```python
from build123d import *

# Parameters (mm, degrees)
SKETCH1_W           = 70.58
SKETCH1_H           = 55.34
SKETCH1_R           = 1.5875
BOSS_EXTRUDE1_DEPTH = 4
SKETCH2_R           = 2.5
CUT_EXTRUDE1_DEPTH  = 6
SKETCH3_R           = 2.5875
SKETCH3_R_2         = 1.5875
SKETCH3_R_3         = 0.9525
BOSS_EXTRUDE2_DEPTH = 3.175


with BuildPart() as part:
    # Sketch1 → Boss-Extrude1 (new, symmetric)
    with BuildSketch(Plane.XY):
        Rectangle(SKETCH1_W, SKETCH1_H)
        with Locations((-20.32, 24.13)):
            Circle(SKETCH1_R, mode=Mode.SUBTRACT)
        with Locations((30.48, 8.89)):
            Circle(SKETCH1_R, mode=Mode.SUBTRACT)
        with Locations((30.48, -19.05)):
            Circle(SKETCH1_R, mode=Mode.SUBTRACT)
        with Locations((-21.59, -24.13)):
            Circle(SKETCH1_R, mode=Mode.SUBTRACT)
    extrude(amount=BOSS_EXTRUDE1_DEPTH, both=True)

    # Sketch2 → Cut-Extrude1 (cut)
    with BuildSketch(Plane(origin=(0, -27.67, 0), x_dir=(1, 0, 0), z_dir=(0, 1, 0))):
        with Locations(Location((30, 0, 0), (0, 0, 270))):
            Circle(SKETCH2_R)
        with Locations(Location((-30, 0, 0), (0, 0, 90))):
            Circle(SKETCH2_R)
    extrude(amount=CUT_EXTRUDE1_DEPTH, mode=Mode.SUBTRACT)

    # Sketch3 → Boss-Extrude2 (add)
    # profile 1 of 4: a face of its own
    with BuildSketch(Plane.XY.offset(4)):
        with Locations(Location((-20.32, 24.13, 0), (0, 0, 180))):
            Circle(SKETCH3_R)
        with Locations((-20.32, 24.13)):
            Circle(SKETCH3_R_2, mode=Mode.SUBTRACT)
    # profile 2 of 4: a face of its own
    with BuildSketch(Plane.XY.offset(4)):
        with Locations(Location((-21.59, -24.13, 0), (0, 0, 180))):
            Circle(SKETCH3_R)
        with Locations((-21.59, -24.13)):
            Circle(SKETCH3_R_3, mode=Mode.SUBTRACT)
    # profile 3 of 4: a face of its own
    with BuildSketch(Plane.XY.offset(4)):
        with Locations(Location((30.48, 8.89, 0), (0, 0, 180))):
            Circle(SKETCH3_R)
        with Locations((30.48, 8.89)):
            Circle(SKETCH3_R_2, mode=Mode.SUBTRACT)
    # profile 4 of 4: a face of its own
    with BuildSketch(Plane.XY.offset(4)):
        with Locations(Location((30.48, -19.05, 0), (0, 0, 180))):
            Circle(SKETCH3_R)
        with Locations((30.48, -19.05)):
            Circle(SKETCH3_R_2, mode=Mode.SUBTRACT)
    extrude(amount=BOSS_EXTRUDE2_DEPTH)


solid = part.part
```
The model under review builds one solid part; all positions refer to its coordinate system, in mm. A direction names the side the tool comes from. Round coordinates to 2 decimals unless told otherwise and drop trailing zeros. Order: outer loops, then holes, each group sorted by start corner. A loop starts at its lowest first (then second) coordinate and runs counter-clockwise, first axis right, second up.
Item 1: Draft analysis for pull direction Z (two halves, no side actions). For faces 1 (the flat face through (0, 0, 4)), 2 (the cylindrical face through (-32.11, -24.71, -1.34)), 3 (the cylindrical face through (31.994, -18.573, 1.509)), 4 (the flat face through (30, -21.67, 0)), state which applies: released by +Z, released by -Z, zero draft, split by the parting line, or undercut.
Working result:
face 1: released by +Z
face 2: undercut
face 3: zero draft
face 4: undercut
Item 2: Add section A-A, the plane y = -24.13. State the section outline as (x, z) points (1 decimal).
Working result:
outline: (-35.3, -4) - (-23.2, -4) - (-23.2, 4) - (-22.5, 4) - (-22.5, 7.2) - (-24.2, 7.2) - (-24.2, 4) - (-35.3, 4) - close; (-20.6, 4) - (-20, 4) - (-20, -4) - (35.3, -4) - (35.3, 4) - (-19, 4) - (-19, 7.2) - (-20.6, 7.2) - close; hole circle Ø5 at (-30, 0); hole circle Ø5 at (30, 0)
Item 3: To check wall thickness, follow probe 1 along Y at (x, z) = (30.48, -1); probe 2 along Z at (x, y) = (-30, -26.3); probe 3 along Y at (x, z) = (-20.32, 3.5). State the ranges of each line that lie inside material, in increasing order.
Working result:
probe 1: y = -21.67 to -20.64, -17.46 to 7.3, 10.48 to 27.67
probe 2: z = -4 to -2.5, 2.5 to 4
probe 3: y = -27.67 to -25.08, -23.18 to 22.54, 25.72 to 27.67
Item 4: For pin 1 (5 mm diameter, centred on x = -1, y = -13.5, fed in from +Z); pin 2 (1.6 mm diameter, centred on x = -21.5, y = -23.5, fed in from -Z), all flat-tipped, find the tip position at first contact; note any pin that passes through.
Working result:
pin 1: stops at z = 4
pin 2: stops at z = 4
Item 5: Add section B-B, the plane z = 0. Count the separate pieces of the cut face and the enclosed holes in it, and give its area (3 significant figures).
Working result:
separate pieces: 1
enclosed holes: 4
area: 3,810 mm2
Item 6: Add section D-D, the plane x = 30. State the section outline as (y, z) points (3 decimals).
Working result:
outline: (-27.67, -4) - (-20.563, -4) - (-20.563, 7.175) - (-21.593, 7.175) - (-21.593, 4) - (-27.67, 4) - (-27.67, 2.5) - (-21.67, 2.5) - (-21.67, -2.5) - (-27.67, -2.5) - close; (-17.537, -4) - (7.377, -4) - (7.377, 7.175) - (6.347, 7.175) - (6.347, 4) - (-16.507, 4) - (-16.507, 7.175) - (-17.537, 7.175) - close; (10.403, -4) - (27.67, -4) - (27.67, 4) - (11.433, 4) - (11.433, 7.175) - (10.403, 7.175) - close
Item 7: Add section C-C, the plane x = -30. State the section outline as (y, z) points.
Working result:
outline: (-27.67, -4) - (27.67, -4) - (27.67, 4) - (-27.67, 4) - (-27.67, 2.5) - (-21.67, 2.5) - (-21.67, -2.5) - (-27.67, -2.5) - close
Item 8: Machinability: for faces 5 (the flat face through (35.29, 0, 0)), 6 (the cylindrical face through (-22.784, -21.834, 5.565)), 7 (the flat face through (-30, -21.67, 0)), 8 (the cylindrical face through (-20.74, -22.79, -0.06)), which of the approach directions +Z, -Z, +X, -X, +Y, -Y give a long, thin tool a straight path to every point of the face, cutting with its end or side? Answer none if there is none.
Working result:
face 5: +Z, -Z, +X, +Y, -Y
face 6: +Z
face 7: -Y
face 8: -Z
